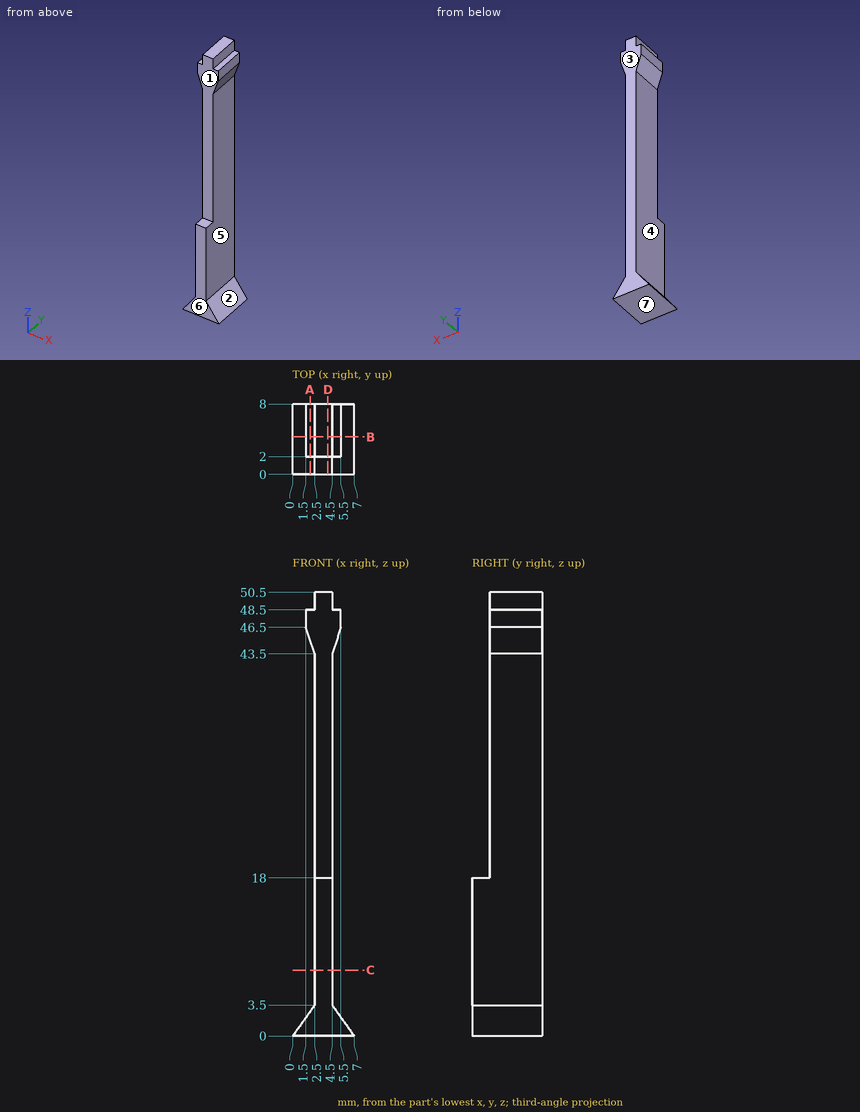
Print and shaded views of the part. All mm, measured from the part's lowest x, y and z. A direction names the side the tool comes from. Round coordinates to 2 decimals unless told otherwise and drop trailing zeros. Loops run counter-clockwise (first coordinate to the right, second up) from the corner with the lowest first, then second, coordinate; pieces in that order, holes last. Notation, with made-up numbers: (52, -4.75) -> (107, -4.75) arc R30 cw to (107, 21.25) -> close; hole circle Ø10 at (64.25, 77.25). An arc over 180 degrees is marked (long way). Use CSV: the item, a comma, the result in double quotes. Start each with the question number.
1) Cut at C-C, the plane z = 7.5. Write the cut outline in (x, y).
2) Wall check: L1, parallel to X at y = 7.25, z = 19; L2, parallel to Y at x = 3.25, z = 27.5; L3, parallel to Z at x = 0.5, y = 5.75. Give the ranges that are in metal, low to high. Write a range as [from, to].
3) Cut at B-B, the plane y = 4.25. Write the cut outline in (x, z).
4) Cut at D-D, the plane x = 4. Write the cut outline in (y, z).
5) Which spindle directions (+Z, -Z, +X, -X, +Y, -Y) get a long thin tool onto all of the face, cutting with end or side? Do the marked faces 1, 2, 3 and 4. Say none if no direction does.
6) Pull direction Z, two halves, no side cores. Call the marked faces 5, 6 and 7: +Z half, -Z half, draft (parallel to the pull), parting line (faces both ways), or undercut.
7) Cut at A-A, the plane x = 2. Write the cut outline in (y, z).
8) Drop flat-ended pins along their axis: P1, Ø0.8, axis at x = 5, y = 5.5, coming from the +Z side; P2, Ø2, axis at x = 3.5, z = 40.5, coming from the -Y side; P3, Ø0.6, axis at y = 5.5, z = 49.5, coming from the +X side; P4, Ø1, axis at x = 5.5, z = 42.5, coming from the -Y side. Give the stop position or say it passes through.
Determined:
1,outline,"(2.5, 0) -> (4.5, 0) -> (4.5, 8) -> (2.5, 8) -> close"
2,L1,"x = [2.5, 4.5]"
2,L2,"y = [2, 8]"
2,L3,"z = [0, 0.7]"
3,outline,"(0, 0) -> (7, 0) -> (4.5, 3.5) -> (4.5, 43.5) -> (5.5, 46.5) -> (5.5, 48.5) -> (4.5, 48.5) -> (4.5, 50.5) -> (2.5, 50.5) -> (2.5, 48.5) -> (1.5, 48.5) -> (1.5, 46.5) -> (2.5, 43.5) -> (2.5, 3.5) -> close"
4,outline,"(0, 0) -> (8, 0) -> (8, 50.5) -> (2, 50.5) -> (2, 18) -> (0, 18) -> close"
5,face 1,"+Z, +X, -X, -Y"
5,face 2,"+X, +Y, -Y"
5,face 3,"+Z, -Z, +X, -X, +Y"
5,face 4,"-X, +Y, -Y"
6,face 5,"undercut"
6,face 6,"draft"
6,face 7,"-Z half"
7,outline,"(0, 0) -> (8, 0) -> (8, 2.8) -> (0, 2.8) -> close; (2, 45) -> (8, 45) -> (8, 48.5) -> (2, 48.5) -> close"
8,P1,"stops at z = 48.5"
8,P2,"stops at y = 2"
8,P3,"stops at x = 4.5"
8,P4,"passes through"
